The listing builds one solid part. Answer for the finished solid, in the listing's coordinates (mm). A direction names the side the tool comes from. Give positions to 0.01 mm unless a question says otherwise; leave off trailing zeros. Write each loop counter-clockwise with the first axis right and the second up, starting at its lowest first coordinate (ties: lowest second). Pieces come first, ordered by that corner, then holes. Notation, with made-up numbers: (-7.5, 66) - (21.5, 66) arc R26 cw to (21.5, 101) - close; hole circle Ø2 at (26.25, -17.5). An arc over 180 degrees is marked (long way). Return JSON: item names as keys, results as strings.
from build123d import *

# Parameters (mm, degrees)
BOSS_EXTRU_3_DEPTH = 3
CONG_2_R           = 70


with BuildPart() as part:
    # Esquisse3 → Boss.-Extru.3 (new body)
    with BuildSketch(Plane.XY):
        Polygon((-52.277721614, 1.004022038), (29.829851332, -13.926203114), (70.552829187, -78.926203114), (70.552829187, -13.926203114), (79.552829187, -13.926203114), (79.552829187, -78.926203114), (120.275807042, -13.926203114), (202.383379989, 1.004022038), (245.052829187, 223.873796886), (210.825087382, 223.873796886), (147.229762937, 36.664572693), (2.875895437, 36.664572693), (-60.719429007, 223.873796886), (-94.947170813, 223.873796886), align=None)
    extrude(amount=BOSS_EXTRU_3_DEPTH)

    # Congé2
    cong_2_edges = [part.edges().sort_by_distance(p)[0] for p in [
        (202.383379989, 1.004022038, 1.5),
        (120.275807042, -13.926203114, 1.5),
        (29.829851332, -13.926203114, 1.5),
        (-52.277721614, 1.004022038, 1.5),
    ]]
    fillet(cong_2_edges, radius=CONG_2_R)


solid = part.part
Item 1: A cutting plane is placed at D-D on x = 54.5. Determine the outline of the cut face in (y, z).
Answer below:
{"outline": "(-53.3, 0) - (36.66, 0) - (36.66, 3) - (-53.3, 3) - close"}
Item 2: A cutting plane is placed at C-C on y = 122.5. Determine the outline of the cut face in (x, z).
Answer below:
{"outline": "(-75.54, 0) - (-26.28, 0) - (-26.28, 3) - (-75.54, 3) - close; (176.39, 0) - (225.64, 0) - (225.64, 3) - (176.39, 3) - close"}
Item 3: For faces 1 (the face through (179.473, 131.58, 1.479)), 2 (the face through (87, 28, 0)), determine the directions among +Z, -Z, +X, -X, +Y, -Y from which every point of the face is accessible in a straight line to the end or side of a thin tool.
Answer below:
{"face 1": "+Z, -Z, +Y", "face 2": "-Z, +X, -X, +Y, -Y"}
Item 4: The mould has two halves that part along X. Classify faces 3 (the face through (-28.477, 128.959, 1.479)), 4 (the face through (58.22, -59.24, 1.48)), 5 (the face through (87, 28, 3)), 6 (the face through (228, 134.8, 1.5)): +X half, -X half, draft (parallel to the pull), parting line (faces both ways), or undercut.
Answer below:
{"face 3": "undercut", "face 4": "-X half", "face 5": "draft", "face 6": "+X half"}
Item 5: A cutting plane is placed at A-A on y = -34. Determine the outline of the cut face in (x, z).
Answer below:
{"outline": "(41.94, 0) - (70.55, 0) - (70.55, 3) - (41.94, 3) - close; (79.55, 0) - (108.17, 0) - (108.17, 3) - (79.55, 3) - close"}
Item 6: Consider L1, parallel to X at y = 140, z = 2.5; L2, parallel to X at y = 128.5, z = 1.8; L3, parallel to Y at x = 117, z = 2.05. Determine where each line is inside the solid, lowest interval first.
Answer below:
{"L1": "x = -78.89 to -32.23, 182.33 to 228.99", "L2": "x = -76.69 to -28.32, 178.43 to 226.79", "L3": "y = -24.68 to 36.66"}
Item 7: Flat-ended cylindrical pins translate along their axes: P1, Ø1, axis at x = 177.5, y = 102.5, coming from the -Z side; P2, Ø0.9, axis at x = 45, z = 1, coming from the +Y side; P3, Ø1, axis at y = 26.5, z = 0.5, coming from the +X side; P4, Ø1.5, axis at y = 134, z = 1.5, coming from the +X side. Find the tip coordinate at first contact, or state that the pin passes through.
Answer below:
{"P1": "stops at z = 0", "P2": "stops at y = 36.66", "P3": "stops at x = 203.68", "P4": "stops at x = 227.99"}
Item 8: A cutting plane is placed at B-B on z = 2.3. Determine the outline of the cut face in (x, y), then the cut area to 3 significant figures.
Answer below:
{"outline": "(-94.95, 223.87) - (-61.3, 48.13) arc R70 ccw to (-5.07, -7.58) - (-0.56, -8.4) arc R70 cw to (46.23, -40.11) - (70.55, -78.93) - (70.55, -13.93) - (79.55, -13.93) - (79.55, -78.93) - (103.87, -40.11) arc R70 cw to (150.67, -8.4) - (155.18, -7.58) arc R70 ccw to (211.41, 48.13) - (245.05, 223.87) - (210.83, 223.87) - (147.23, 36.66) - (2.88, 36.66) - (-60.72, 223.87) - close", "area": "32,000 mm²"}
